from build123d import *

# Parameters (mm, degrees)
F0_W      = 100
F0_H      = 110
F1_DEPTH  = 6
F2_W      = 10
F2_H      = 5
F3_DEPTH  = 6.001
F5_R      = 3.8
F5_R_2    = 2.6
F6_DEPTH  = 6.001
F7_DEPTH  = 13.5
F10_DEPTH = 13.5
F12_DEPTH = 3
F14_DEPTH = 3
F16_DEPTH = 3
F17_R     = 1.75
F18_DEPTH = 82.3823972081
F19_R     = 1.75
F20_DEPTH = 82.3823972081
F21_R     = 1.5
F22_R     = 10
F24_DEPTH = 3
F25_R     = 3
F26_R     = 1.75
F27_DEPTH = 59.751


with BuildPart() as f1:
    # F0 (on Top) → F1 (new body)
    with BuildSketch(Plane.XY):
        Rectangle(F0_W, F0_H)
    extrude(amount=F1_DEPTH)

    # F2 (on face) → F3 (cut, through all)
    with BuildSketch(Plane.XY.offset(6)):
        with Locations((0, 47.5)):
            Rectangle(F2_W, F2_H)
        with Locations((0, -47.5)):
            Rectangle(F2_W, F2_H)
    extrude(amount=-F3_DEPTH, mode=Mode.SUBTRACT)

    # F5 (on face) → F6 (cut, through all)
    with BuildSketch(Plane.XY.offset(6)):
        with Locations((21, -40)):
            Circle(F5_R)
        with Locations((21, 40)):
            Circle(F5_R)
        with Locations((-21, 40)):
            Circle(F5_R_2)
        with Locations((-21, -40)):
            Circle(F5_R_2)
    extrude(amount=-F6_DEPTH, mode=Mode.SUBTRACT)

    # F4 (on face) → F7 (join)
    with BuildSketch(Plane.XY.offset(6)):
        Polygon((50, 21.0732848254), (0, -7.7942286341), (-50, 21.0732848254), (-50, 17.6091832103), (-9.75, -5.6291651246), (-9.75, -55), (-6.75, -55), (-6.75, -7.3612159322), (0, -11.2583302492), (6.75, -7.3612159322), (6.75, -55), (9.75, -55), (9.75, -5.6291651246), (50, 17.6091832103), align=None)
        Polygon((-50, 36.6617420935), (0, 7.7942286341), (50, 36.6617420935), (50, 40.1258437087), (0, 11.2583302492), (-50, 40.1258437087), align=None)
    extrude(amount=F7_DEPTH)

    # F9 (on face) → F10 (join)
    with BuildSketch(Plane.XY.offset(19.5)):
        Polygon((-9.75, 16.8874953738), (-9.75, -55), (-6.75, -55), (-6.75, 15.1554445662), align=None)
        Polygon((9.75, 16.8874953738), (6.75, 15.1554445662), (6.75, -55), (9.75, -55), align=None)
    extrude(amount=F10_DEPTH)

    # F11 (on face) → F12 (join)
    with BuildSketch(Plane.XY.offset(19.5)):
        Polygon((9.75, 16.8874953738), (9.75, -5.6291651246), (50, 17.6091832103), (50, 40.1258437087), align=None)
        Polygon((-50, 40.1258437087), (-50, 17.6091832103), (-9.75, -5.6291651246), (-9.75, 16.8874953738), align=None)
    extrude(amount=F12_DEPTH)

    # F13 (on offset) → F14 (join)
    with BuildSketch(Plane.XY.offset(19.5)):
        Polygon((-6.75, -7.3612159322), (-6.75, -55), (6.75, -55), (6.75, -7.3612159322), (0, -11.2583302492), align=None)
    extrude(amount=-F14_DEPTH)

    # F15 (on face) → F16 (join)
    with BuildSketch(Plane.XY.offset(33)):
        Polygon((0, 11.2583302492), (-9.75, 16.8874953738), (-9.75, -55), (9.75, -55), (9.75, 16.8874953738), align=None)
    extrude(amount=F16_DEPTH)

    # F17 (on face) → F18 (cut, through all)
    with BuildSketch(Plane(origin=(4.875, -8.4437476869, 0), x_dir=(0.8660254038, 0.5, 0), z_dir=(0.5, -0.8660254038, 0))):
        with Locations((32.1058617944, 12.75)):
            Circle(F17_R)
    extrude(amount=-F18_DEPTH, mode=Mode.SUBTRACT)

    # F19 (on face) → F20 (cut, through all)
    with BuildSketch(Plane(origin=(-4.875, -8.4437476869, 0), x_dir=(0.8660254038, -0.5, 0), z_dir=(-0.5, -0.8660254038, 0))):
        with Locations((-32.1058617944, 12.75)):
            Circle(F19_R)
    extrude(amount=-F20_DEPTH, mode=Mode.SUBTRACT)

    # F21
    f21_edges = [f1.edges().sort_by_distance(p)[0] for p in [
        (0, 50, 6),
        (0, 50, 0),
        (0, -50, 0),
        (0, -50, 6),
    ]]
    fillet(f21_edges, radius=F21_R)

    # F22
    f22_edges = [f1.edges().sort_by_distance(p)[0] for p in [
        (-50, -55, 3),
        (50, -55, 3),
        (50, 55, 3),
        (-50, 55, 3),
    ]]
    fillet(f22_edges, radius=F22_R)

    # F23 (on face) → F24 (join)
    with BuildSketch(Plane.XZ.offset(55)):
        Polygon((-9.75, 6), (-9.75, 36), (-40, 6), align=None)
        Polygon((9.75, 6), (40, 6), (9.75, 36), align=None)
    extrude(amount=-F24_DEPTH)

    # F25
    f25_edges = [f1.edges().sort_by_distance(p)[0] for p in [
        (-9.75, 5.629165, 22.5),
        (-9.75, -28.814583, 6),
        (-9.75, -5.629165, 14.25),
        (-29.875, 5.990009, 6),
        (9.75, -28.814583, 6),
        (9.75, -5.629165, 14.25),
        (9.75, 5.629165, 22.5),
        (29.875, 5.990009, 6),
        (24.875, -52, 6),
        (-24.875, -52, 6),
        (25, 25.692087, 6),
        (-25, 25.692087, 6),
        (0, 11.25833, 12.75),
        (9.75, -52, 21),
        (-9.75, -52, 21),
    ]]
    fillet(f25_edges, radius=F25_R)

    # F26 (on face) → F27 (cut, through all)
    with BuildSketch(Plane.YZ.offset(9.75)):
        with Locations((-15, 26.25)):
            Circle(F26_R)
    extrude(amount=-F27_DEPTH, mode=Mode.SUBTRACT)


solid = f1.part
Geometry check sheet. Reference: the model listing, model coordinates, mm. A direction names the side the tool comes from. Give positions to 0.01 mm unless a question says otherwise; leave off trailing zeros. Order: outer loops, then holes, each group sorted by start corner. A loop starts at its lowest first (then second) coordinate and runs counter-clockwise, first axis right, second up. Notation, with made-up numbers: (-23.75, 16) - (30.25, 16) arc R23 cw to (30.25, 51) - close; hole circle Ø11 at (10, 88.25). An arc over 180 degrees is marked (long way). Use one line per item in the form item = value.
1) Material ranges on probe 1 along Y at (x, z) = (21, 4.1); probe 2 along X at (y, z) = (-17, 9.5), recorded low to high. Write a range as from..to.
Working result:
probe_1 = -55..-43.8, -36.2..36.2, 43.8..55
probe_2 = -9.75..-6.75, 6.75..9.75
2) Sectioned sample at B-B (y = -15). Record the boundary of the cut face in (x, z), and give its area (3 significant figures).
Working result:
outline = (-50, 0) - (50, 0) - (50, 6) - (12.75, 6) arc R3 cw to (9.75, 9) - (9.75, 24.5) - (6.75, 24.5) - (6.75, 19.5) - (-6.75, 19.5) - (-6.75, 24.5) - (-9.75, 24.5) - (-9.75, 9) arc R3 cw to (-12.75, 6) - (-50, 6) - close; (-9.75, 28) - (-6.75, 28) - (-6.75, 33) - (6.75, 33) - (6.75, 28) - (9.75, 28) - (9.75, 36) - (-9.75, 36) - close; hole (-6.75, 6) - (6.75, 6) - (6.75, 16.5) - (-6.75, 16.5) - close
area = 844 mm^2
3) Access from +Z, -Z, +X, -X, +Y, -Y to the whole of each face (thin tool, end or side, straight path). Record for faces 1 (the face through (-10.65, -28.47, 6.86)), 2 (the face through (0, -31, 16.5)), 3 (the face through (9.75, -24, 22)).
Working result:
face_1 = +Z, -X
face_2 = -Y
face_3 = +Z, +X
4) Depth check by flat-ended pin: pin 1 Ø1 at (x, z) = (-12, 27.5) entering from +Y; pin 2 Ø8 at (y, z) = (-3.5, 17.5) entering from +X; pin 3 Ø3 at (y, z) = (-15, 26.25) entering from -X; pin 4 Ø8 at (x, y) = (0.5, 13) entering from +Z. Enter the tip coordinate at first touch or a pass-through.
Working result:
pin_1 = -51.73
pin_2 = 20.37
pin_3 = through
pin_4 = 36
5) Draft check along Y on faces 4 (the face through (-5, -48, 3)), 5 (the face through (19, -52, 16)), 6 (the face through (-50, 9, 4)), 7 (the face through (-0.022, 11.723, 14.324)). Enter one of: released by +Y, released by -Y, zero draft, split by the parting line, or undercut.
Working result:
face_4 = undercut
face_5 = undercut
face_6 = zero draft
face_7 = released by +Y
6) Sectioned sample at A-A (y = -40). Record the boundary of the cut face in (x, z).
Working result:
outline = (-50, 0) - (-23.6, 0) - (-23.6, 6) - (-50, 6) - close; (-18.4, 0) - (17.2, 0) - (17.2, 6) - (12.75, 6) arc R3 cw to (9.75, 9) - (9.75, 36) - (-9.75, 36) - (-9.75, 9) arc R3 cw to (-12.75, 6) - (-18.4, 6) - close; (24.8, 0) - (50, 0) - (50, 6) - (24.8, 6) - close; hole (-6.75, 6) - (6.75, 6) - (6.75, 16.5) - (-6.75, 16.5) - close; hole (-6.75, 19.5) - (6.75, 19.5) - (6.75, 33) - (-6.75, 33) - close
